Model file for the job. Use its own axes, mm. Face numbers are marked on the shaded views. A direction names the side the tool comes from. Give positions to 0.01 mm unless a question says otherwise; leave off trailing zeros. Loops run counter-clockwise (first coordinate to the right, second up) from the corner with the lowest first, then second, coordinate; pieces in that order, holes last. Notation, with made-up numbers: (19.5, 37.5) -> (58.5, 37.5) arc R15 ccw to (58.5, 55.5) -> close; hole circle Ø9 at (-31, -24.5). An arc over 180 degrees is marked (long way). Use CSV: the item, a comma, the result in double quotes. Start each with the question number.
(1) Drill centre lines: probe 1 along X at (y, z) = (33, 5.5); probe 2 along Y at (x, z) = (54, 9). Where is each one in solid material? Low to high.
(2) Cut at C-C on y = 8. Write the cut outline in (x, z), then the cut area to 3 significant figures.
(3) Cut at B-B on z = -9.5. Write the cut outline in (x, y), then the cut area to 3 significant figures.
(4) 3-axis set-ups, long thin cutter, end or side, ignore diameter. For the marked faces 1, 2, 3, 4 and 5: which of +Z, -Z, +X, -X, +Y, -Y reach the whole face in a straight line?
(5) Pull direction Y, two halves, no side cores. Call the marked faces 6, 7 and 8: pulls with the +Y half, pulls with the -Y half, needs draft (parallel to the pull), parting line crosses it, or undercut.
(6) Cut at D-D on x = 118. Write the cut outline in (y, z).
(7) Cut at A-A on x = 1. Write the cut outline in (y, z), then the cut area to 3 significant figures.
(8) Flat gauge pins, fed straight in: pin 1 (10 mm diameter, centred on x = 46, z = -24, fed in from -Y); pin 2 (12 mm diameter, centred on x = 61.5, y = 23, fed in from -Z); pin 3 (20 mm diameter, centred on x = 62.5, y = 25, fed in from +Z). Where does each tip first touch, or does it go through?
from build123d import *

# Parameters (mm, degrees)
SKETCH1_W           = 65
SKETCH1_H           = 65
SKETCH1_W_2         = 25
SKETCH1_H_2         = 25
BOSS_EXTRUDE1_DEPTH = 50
SKETCH2_W           = 40
SKETCH2_H           = 40
SKETCH2_W_2         = 30
SKETCH2_H_2         = 30
BOSS_EXTRUDE2_DEPTH = 100


with BuildPart() as part:
    # Sketch1 → Boss-Extrude1 (new body)
    with BuildSketch(Plane(origin=(0, 0, 0), x_dir=(1, 0, 0), z_dir=(0, 1, 0))):
        Rectangle(SKETCH1_W, SKETCH1_H)
        Rectangle(SKETCH1_W_2, SKETCH1_H_2, mode=Mode.SUBTRACT)
    extrude(amount=BOSS_EXTRUDE1_DEPTH)

    # Sketch2 → Boss-Extrude2 (add)
    with BuildSketch(Plane(origin=(32.5, 0, 0), x_dir=(0, 0, -1), z_dir=(1, 0, 0))):
        with Locations((0, 25)):
            Rectangle(SKETCH2_W, SKETCH2_H)
        with Locations((0, 25)):
            Rectangle(SKETCH2_W_2, SKETCH2_H_2, mode=Mode.SUBTRACT)
    extrude(amount=BOSS_EXTRUDE2_DEPTH)


solid = part.part
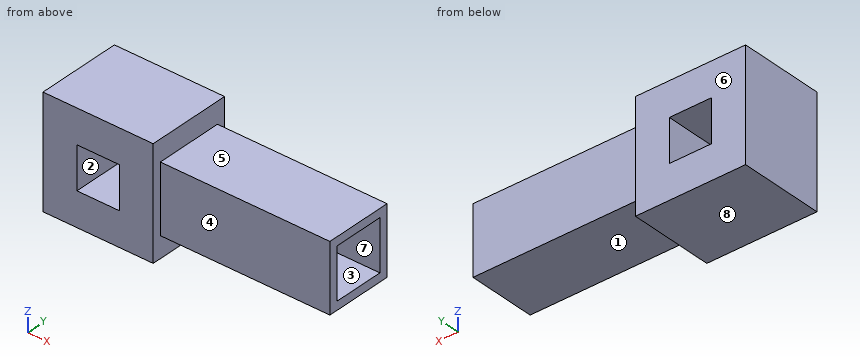
Check result:
1,probe 1,"-32.5 to -12.5, 12.5 to 32.5"
1,probe 2,"5 to 10, 40 to 45"
2,outline,"(-32.5, -32.5) -> (32.5, -32.5) -> (32.5, -20) -> (132.5, -20) -> (132.5, 20) -> (32.5, 20) -> (32.5, 32.5) -> (-32.5, 32.5) -> close; hole (-12.5, -12.5) -> (12.5, -12.5) -> (12.5, 12.5) -> (-12.5, 12.5) -> close"
2,area,"7,600 mm²"
3,outline,"(-32.5, 0) -> (-12.5, 0) -> (-12.5, 50) -> (-32.5, 50) -> close; (12.5, 0) -> (32.5, 0) -> (32.5, 5) -> (132.5, 5) -> (132.5, 10) -> (32.5, 10) -> (32.5, 40) -> (132.5, 40) -> (132.5, 45) -> (32.5, 45) -> (32.5, 50) -> (12.5, 50) -> close"
3,area,"3,000 mm²"
4,face 1,"-Z, +X, +Y, -Y"
4,face 2,"+Y, -Y"
4,face 3,"+X"
4,face 4,"+Z, -Z, +X, -Y"
4,face 5,"+Z, +X, +Y, -Y"
5,face 6,"pulls with the +Y half"
5,face 7,"undercut"
5,face 8,"needs draft"
6,outline,"(5, -20) -> (45, -20) -> (45, 20) -> (5, 20) -> close; hole (10, -15) -> (40, -15) -> (40, 15) -> (10, 15) -> close"
7,outline,"(0, -32.5) -> (50, -32.5) -> (50, -12.5) -> (0, -12.5) -> close; (0, 12.5) -> (50, 12.5) -> (50, 32.5) -> (0, 32.5) -> close"
7,area,"2,000 mm²"
8,pin 1,"y = 5"
8,pin 2,"z = -20"
8,pin 3,"z = 20"
